Source: CAD feature listing. Evaluate the final solid. Frame: model axes, mm. A direction names the side the tool comes from. Round coordinates to 2 decimals unless told otherwise and drop trailing zeros. Order: outer loops, then holes, each group sorted by start corner. A loop starts at its lowest first (then second) coordinate and runs counter-clockwise, first axis right, second up. Notation, with made-up numbers: (-13, -36.5) -> (28, -36.5) arc R4 cw to (28, -30.5) -> close; hole circle Ø2 at (69, 86.5). An arc over 180 degrees is marked (long way). One line per item, written item: value. Start each with the question number.
1) Section A-A (z = 15.5). Return the cut outline in (x, y).
2) Section C-C (x = 0). Return the cut outline in (y, z), and give its area (3 significant figures).
3) Pin query (flat end, axial travel): P1, Ø5, axis at y = 29, z = 61, coming from the +X side; P2, Ø1.5, axis at x = -19.5, z = 65.5, coming from the +Y side; P3, Ø12, axis at y = 20, z = 48.5, coming from the -X side; P4, Ø0.6, axis at y = -31, z = 55.5, coming from the -X side. Return the tip coordinate at first contact, or that it passes through.
4) Section D-D (z = 47). Return the cut outline in (x, y).
5) Ray query, L1, parallel to Y at x = 0, z = 1.3; L2, parallel to X at y = 38, z = 1 (3 decimals); L3, parallel to Y at x = -18, z = 72. Return the intervals inside material, ascending.
6) Reachability of faces 5 (the face through (-20.608, 26.044, 46.37)), 6 (the face through (-19.868, 28, 36)), 7 (the face through (-21.368, 30, 36)), 8 (the face through (-16.368, -33, 46)), 9 (the face through (0.85, 39.44, 0.99)) from +Z, -Z, +X, -X, +Y, -Y: full face, straight path, thin tool, end or side. Return the list, or none.
7) Mould query, pull axis Y, two halves, no side actions, for faces 1 (the face through (-19, -33, 92)), 2 (the face through (-19, -35.1, 46)), 3 (the face through (-19, 35.1, 46)), 4 (the face through (-0.34, -39.65, 0.99)). Classes: pulls with the +Y half, pulls with the -Y half, needs draft (parallel to the pull), parting line crosses it, or undercut.
8) Section B-B (y = 38.1). Return the cut outline in (x, z) (1 decimal), and give its area (4 significant figures).
```python
from build123d import *

# Parameters (mm, degrees)
FRONT_FACE_W        = 44.45
FRONT_FACE_H        = 88.9
FRONT_FACE_R        = 1.5875
BOSS_EXTRUDE1_DEPTH = 2
CANTIARM_W          = 90
CANTIARM_H          = 5
BOSS_EXTRUDE2_DEPTH = 2.5
CHANNEL_W           = 2
CHANNEL_H           = 2
CUT_EXTRUDE1_DEPTH  = 91
BOSS_EXTRUDE5_START = 1
BOSS_EXTRUDE5_DEPTH = 1.5


with BuildPart() as part:
    # Front Face → Boss-Extrude1 (new body)
    with BuildSketch(Plane.XY):
        Rectangle(FRONT_FACE_W, FRONT_FACE_H)
        with Locations((0, 38.1)):
            Circle(FRONT_FACE_R, mode=Mode.SUBTRACT)
        with Locations((0, -38.1)):
            Circle(FRONT_FACE_R, mode=Mode.SUBTRACT)
    extrude(amount=BOSS_EXTRUDE1_DEPTH)

    # CantiArm → Boss-Extrude2 (add, symmetric)
    with BuildSketch(Plane.ZY.offset(18.868316672)):
        with Locations((47, 32.6)):
            Rectangle(CANTIARM_W, CANTIARM_H)
    boss_extrude2 = extrude(amount=BOSS_EXTRUDE2_DEPTH, both=True)

    # Channel → Cut-Extrude1 (cut, through all)
    with BuildSketch(Plane.XY.offset(2)):
        with Locations((-18.868316672, 31.1)):
            Rectangle(CHANNEL_W, CHANNEL_H)
    cut_extrude1 = extrude(amount=CUT_EXTRUDE1_DEPTH, mode=Mode.SUBTRACT)

    # Sketch5 → Boss-Extrude5 (add)
    with BuildSketch(Plane.ZY.offset(18.868316672).offset(BOSS_EXTRUDE5_START)):
        Polygon((2, 22.1), (92, 30.1), (2, 30.1), align=None)
    boss_extrude5 = extrude(amount=BOSS_EXTRUDE5_DEPTH)

    # Mirror1: Boss-Extrude2, Cut-Extrude1, Boss-Extrude5 across plane
    add(boss_extrude2.mirror(Plane.ZX))
    add(cut_extrude1.mirror(Plane.ZX), mode=Mode.SUBTRACT)
    add(boss_extrude5.mirror(Plane.ZX))


solid = part.part
```
Findings:
1. outline: (-21.37, -35.1) -> (-16.37, -35.1) -> (-16.37, -30.1) -> (-17.87, -30.1) -> (-17.87, -32.1) -> (-19.87, -32.1) -> (-19.87, -23.3) -> (-21.37, -23.3) -> close; (-21.37, 23.3) -> (-19.87, 23.3) -> (-19.87, 32.1) -> (-17.87, 32.1) -> (-17.87, 30.1) -> (-16.37, 30.1) -> (-16.37, 35.1) -> (-21.37, 35.1) -> close
2. outline: (-44.45, 0) -> (-39.69, 0) -> (-39.69, 2) -> (-44.45, 2) -> close; (-36.51, 0) -> (36.51, 0) -> (36.51, 2) -> (-36.51, 2) -> close; (39.69, 0) -> (44.45, 0) -> (44.45, 2) -> (39.69, 2) -> close
2. area: 165 mm2
3. P1: x = -16.37
3. P2: y = 35.1
3. P3: through
3. P4: x = -21.37
4. outline: (-21.37, -35.1) -> (-16.37, -35.1) -> (-16.37, -30.1) -> (-17.87, -30.1) -> (-17.87, -32.1) -> (-19.87, -32.1) -> (-19.87, -26.1) -> (-21.37, -26.1) -> close; (-21.37, 26.1) -> (-19.87, 26.1) -> (-19.87, 32.1) -> (-17.87, 32.1) -> (-17.87, 30.1) -> (-16.37, 30.1) -> (-16.37, 35.1) -> (-21.37, 35.1) -> close
5. L1: -44.45 to -39.69, -36.51 to 36.51, 39.69 to 44.45
5. L2: -22.225 to -1.584, 1.584 to 22.225
5. L3: -35.1 to -32.1, 32.1 to 35.1
6. face 5: +Z, +X, -X
6. face 6: +Z
6. face 7: +Z, -X, +Y, -Y
6. face 8: +Z, +X, +Y, -Y
6. face 9: +Z, -Z
7. face 1: needs draft
7. face 2: pulls with the -Y half
7. face 3: pulls with the +Y half
7. face 4: undercut
8. outline: (-22.2, 0) -> (-1.6, 0) -> (-1.6, 2) -> (-22.2, 2) -> close; (1.6, 0) -> (22.2, 0) -> (22.2, 2) -> (1.6, 2) -> close
8. area: 82.55 mm2
